from build123d import *

# Parameters (mm, degrees)
F1_DEPTH = 340
F3_DEPTH = 50
F5_D     = 12


with BuildPart() as f1:
    # F0 (on Front) → F1 (new body, symmetric)
    with BuildSketch(Plane.XZ):
        with BuildLine():
            ThreePointArc((15, 19), (13.2426406871, 23.2426406871), (9, 25))
            Line((9, 25), (-9, 25))
            ThreePointArc((-9, 25), (-13.2426406871, 23.2426406871), (-15, 19))
            Line((-15, 19), (-15, -19))
            ThreePointArc((-15, -19), (-13.2426406871, -23.2426406871), (-9, -25))
            Line((-9, -25), (9, -25))
            ThreePointArc((9, -25), (13.2426406871, -23.2426406871), (15, -19))
            Line((15, -19), (15, 19))
        make_face()
        with BuildLine():
            Line((-9, 22), (9, 22))
            ThreePointArc((9, 22), (11.1213203436, 21.1213203436), (12, 19))
            Line((12, 19), (12, -19))
            ThreePointArc((12, -19), (11.1213203436, -21.1213203436), (9, -22))
            Line((9, -22), (-9, -22))
            ThreePointArc((-9, -22), (-11.1213203436, -21.1213203436), (-12, -19))
            Line((-12, -19), (-12, 19))
            ThreePointArc((-12, 19), (-11.1213203436, 21.1213203436), (-9, 22))
        make_face(mode=Mode.SUBTRACT)
    extrude(amount=F1_DEPTH, both=True)

    # F2 (on face) → F3 (cut, through all)
    with BuildSketch(Plane.XY.offset(25)):
        Polygon((-9, -340), (-9, -334), (-15, -340), align=None)
        Polygon((9, -340), (9, -316), (-9, -334), (-9, -340), align=None)
        Polygon((15, -310), (9, -316), (9, -340), (15, -340), align=None)
        Polygon((-15, 340), (-9, 334), (-9, 340), align=None)
        Polygon((-9, 334), (9, 316), (9, 340), (-9, 340), align=None)
        Polygon((9, 316), (15, 310), (15, 340), (9, 340), align=None)
    extrude(amount=-F3_DEPTH, mode=Mode.SUBTRACT)

    # F5 (through all)
    with Locations(Plane(origin=(-15, 0, 0), x_dir=(0, -1, 0), z_dir=(-1, 0, 0))):
        with Locations((-220, 0)):
            Hole(F5_D / 2)


solid = f1.part
The listing builds one solid part. Answer for the finished solid, in the listing's coordinates (mm). A direction names the side the tool comes from. Coordinates: 2 decimals unless noted, no trailing zeros. Loops run counter-clockwise (first coordinate to the right, second up) from the corner with the lowest first, then second, coordinate; pieces in that order, holes last. Notation, with made-up numbers: M 60.5,-3 L 94.5,-3 A21 cw 94.5,35 Z; hole C 32,-3.75 d5. An arc over 180 degrees is marked long. Answer in a Markdown table with one row per item.
1) Which of the six approach directions +Z, -Z, +X, -X, +Y, -Y give full straight-line access (tool end or side, diameter ignored) to faces 4 (the cylindrical face through (13.521, 225.723, 1.802)), 5 (the flat face through (12, -4, 0))?
Answers below:
| item | result |
|---|---|
| face 4 | +X, -X |
| face 5 | +Y, -Y |
2) Find section D-D (y = 220). Determine the outline of the cut face in (x, z), then the cut area to 3 significant figures.
Answers below:
| item | result |
|---|---|
| outline | M -15,-19 A6 ccw -9,-25 L 9,-25 A6 ccw 15,-19 L 15,-6 L 12,-6 L 12,-19 A3 cw 9,-22 L -9,-22 A3 cw -12,-19 L -12,-6 L -15,-6 Z; M -15,6 L -12,6 L -12,19 A3 cw -9,22 L 9,22 A3 cw 12,19 L 12,6 L 15,6 L 15,19 A6 ccw 9,25 L -9,25 A6 ccw -15,19 Z |
| area | 349 mm^2 |
3) Find the intervals of material crossed by probe 1 along Z at (x, y) = (1.25, 33); probe 2 along X at (y, z) = (190.5, -2); probe 3 along X at (y, z) = (-78, 21.5), in increasing order.
Answers below:
| item | result |
|---|---|
| probe 1 | -25 to -22, 22 to 25 |
| probe 2 | -15 to -12, 12 to 15 |
| probe 3 | -14.45 to -10.66, 10.66 to 14.45 |
4) Given pin 1 (14 mm diameter, centred on y = 220, z = 0, fed in from -X); pin 2 (9.5 mm diameter, centred on y = 220, z = 0, fed in from -X), each flat-ended and moving along its own axis, determine where each tip first touches the part or whether it passes through.
Answers below:
| item | result |
|---|---|
| pin 1 | x = -15 |
| pin 2 | through |
5) Find section C-C (y = -237). Determine the outline of the cut face in (x, z), then the cut area to 3 significant figures.
Answers below:
| item | result |
|---|---|
| outline | M -15,-19 A6 ccw -9,-25 L 9,-25 A6 ccw 15,-19 L 15,19 A6 ccw 9,25 L -9,25 A6 ccw -15,19 Z; hole M -12,-19 A3 ccw -9,-22 L 9,-22 A3 ccw 12,-19 L 12,19 A3 ccw 9,22 L -9,22 A3 ccw -12,19 Z |
| area | 421 mm^2 |
6) Find section B-B (z = 0). Determine the outline of the cut face in (x, y).
Answers below:
| item | result |
|---|---|
| outline | M -15,-340 L -12,-337 L -12,214 L -15,214 Z; M -15,226 L -12,226 L -12,337 L -15,340 Z; M 12,-313 L 15,-310 L 15,214 L 12,214 Z; M 12,226 L 15,226 L 15,310 L 12,313 Z |
7) Find section A-A (x = 1.25). Determine the outline of the cut face in (y, z).
Answers below:
| item | result |
|---|---|
| outline | M -323.75,-25 L 323.75,-25 L 323.75,-22 L -323.75,-22 Z; M -323.75,22 L 323.75,22 L 323.75,25 L -323.75,25 Z |
8) Determine the mould class of faces 1 (the flat face through (-12, -5, 0)), 2 (the flat face through (12.3, -312.7, 2)), 3 (the cylindrical face through (-13.479, 225.723, 1.802)) for opening direction Y: released by +Y, released by -Y, zero draft, split by the parting line, or undercut.
Answers below:
| item | result |
|---|---|
| face 1 | zero draft |
| face 2 | released by -Y |
| face 3 | undercut |
